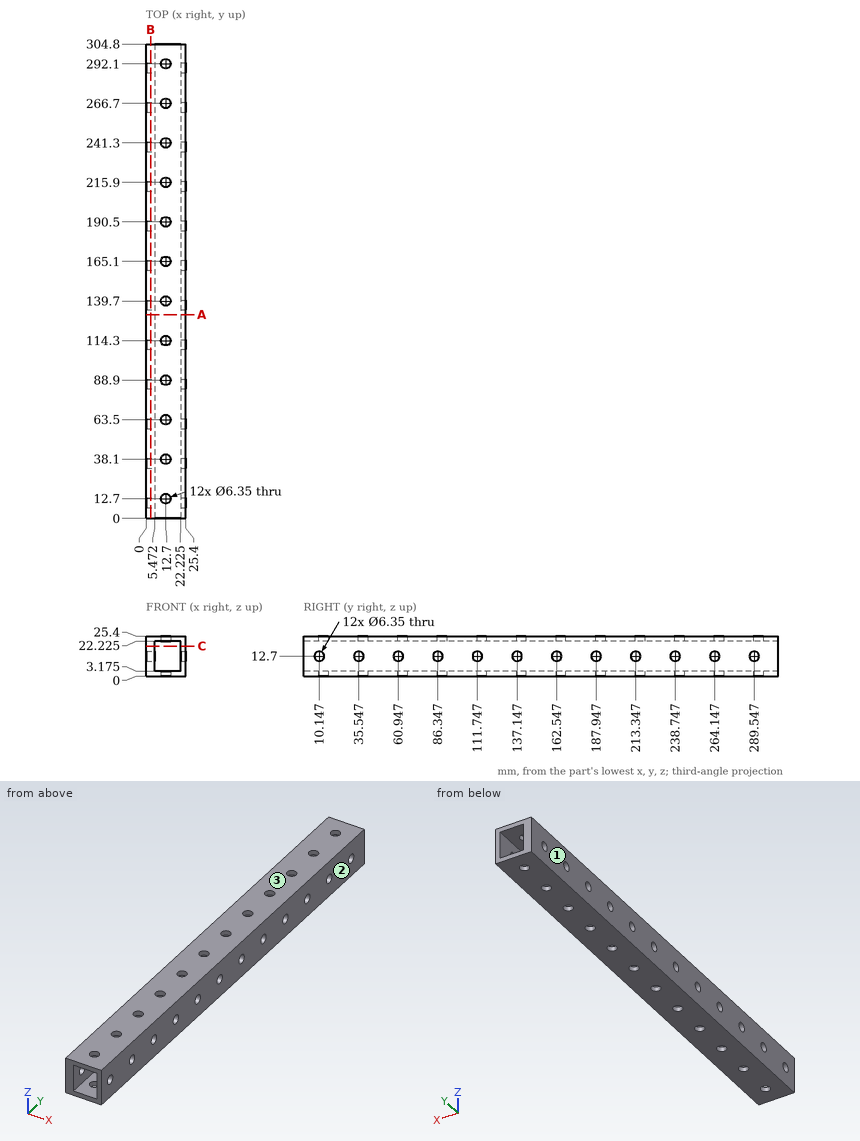
The drawing under review shows one solid part. Ordinate dimensions are in mm from its lowest x, y, z. Give positions to 0.01 mm unless a question says otherwise; leave off trailing zeros. Write each loop counter-clockwise with the first axis right and the second up, starting at its lowest first coordinate (ties: lowest second). Pieces come first, ordered by that corner, then holes.
1. Draft analysis for pull direction X (two halves, no side actions). For the marked faces 1, 2 and 3, state which applies: +X half, -X half, draft (parallel to the pull), parting line (faces both ways), or undercut.
2. Add section B-B, the plane x = 3. Count the separate pieces of the cut face and the enclosed holes in it, plus the area to 3 significant figures.
3. Add section C-C, the plane z = 19.25. Write out the cut boundary in (x, y) (1 decimal).
4. For P1, Ø4, axis at x = 12.7, y = 215.9, coming from the -Z side, flat-tipped, find the tip position at first contact; note if it passes through.
5. Add section A-A, the plane y = 131. Write out the cut boundary in (x, z) (1 decimal), plus the area to 3 significant figures.
6. Wall thickness on L1, parallel to Z at x = 6.75, y = 92.5 (1 decimal); L2, parallel to X at y = 234, z = 5 (1 decimal): over which ranges is each line inside the solid? List them lowest first.
Worked answers:
1. face 1: -X half
1. face 2: +X half
1. face 3: draft
2. separate pieces: 1
2. enclosed holes: 12
2. area: 7,360 mm2
3. outline: (0, 0) - (5.5, 0) - (5.5, 304.8) - (0, 304.8) - close; (22.2, 0) - (25.4, 0) - (25.4, 304.8) - (22.2, 304.8) - close
4. P1: passes through
5. outline: (0, 0) - (25.4, 0) - (25.4, 25.4) - (0, 25.4) - close; hole (5.5, 3.2) - (22.2, 3.2) - (22.2, 22.2) - (5.5, 22.2) - close
5. area: 326 mm2
6. L1: z = 0 to 3.2, 22.2 to 25.4
6. L2: x = 0 to 5.5, 22.2 to 25.4
